Autodesk Inventor part; units mm, degrees
ref_plane "YZ Plane" through (0, 0, 0) normal (1, 0, 0) x (0, 1, 0)
ref_plane "XZ Plane" through (0, 0, 0) normal (0, 1, 0) x (-1, 0, 0)
ref_plane "XY Plane" through (0, 0, 0) normal (0, 0, 1) x (1, 0, 0)
sketch "Sketch1" plane through (0, 0, 0) normal (0, 0, 1) x (1, 0, 0)
  circle A0 centre (0, 0) radius 1.5
  dimension "Diameter" = 3
extrude "Extrusion1" add sketch "Sketch1" along normal blind 48
sketch "Sketch2" plane through (0, 0, 0) normal (0, 0, -1) x (-1, 0, 0)
  circle A0 centre (0, 0) radius 1.5 construction
  circle A1 centre (0, 0) radius 2.25
  dimension "Head_Washer_Diameter" = 4.5
extrude "Extrusion2" add sketch "Sketch2" along normal blind 0.25
sketch "Sketch3" plane through (0, 0, -0.25) normal (0, 0, -1) x (-1, 0, 0)
  circle A0 centre (0, 0) radius 2.25 construction
  line L0 (-2.25, 1.299) -> (0, 2.5981)
  line L1 (0, 2.5981) -> (2.25, 1.299)
  line L2 (2.25, 1.299) -> (2.25, -1.299)
  line L3 (2.25, -1.299) -> (0, -2.5981)
  line L4 (0, -2.5981) -> (-2.25, -1.299)
  line L5 (-2.25, -1.299) -> (-2.25, 1.299)
extrude "Extrusion3" add sketch "Sketch3" along normal blind 2.001
thread "Thread1"
chamfer "Chamfer1" distance 0.25 angle 45 1 edges at (-1.5, 0, 48)
sketch "Sketch4" plane through (0, 0, 0) normal (0, 1, 0) x (-1, 0, 0)
  line L0 (-2.25, -0.25) -> (-2.25, -2.251) construction
  line L1 (-2.25, -0.25) -> (-2.25, -2.251) construction
  line L2 (-2.25, -2.251) -> (-3.45, -2.251)
  line L3 (-3.45, -2.251) -> (-3.45, -1.5582)
  line L4 (-3.45, -1.5582) -> (-2.25, -2.251)
  line L5 (0, 0) -> (0, -6.83)
  point P0 (-2.25, -0.25)
  dimension "Head_Chamfer_Angle" = 30
  dimension "d14" = 1.2
revolve "Revolution1" cut sketch "Sketch4" angle 360 about axis through (0, 0, 0) along (0, 0, -1)
equation "\"Head_Washer_Diameter\" = 1.5 * Diameter"
equation "\"Head_Height\" = 0.667 * Diameter"
equation "\"d14\" = 0.4 * Diameter"
properties part number "Hex Head Cap Screw"
The listing builds one solid part. Answer for the finished solid, in the listing's coordinates (mm). A direction names the side the tool comes from. Round coordinates to 2 decimals unless told otherwise and drop trailing zeros. Order: outer loops, then holes, each group sorted by start corner. A loop starts at its lowest first (then second) coordinate and runs counter-clockwise, first axis right, second up. Notation, with made-up numbers: (-12, -32.75) -> (38, -32.75) arc R31 ccw to (38, -2.75) -> close; hole circle Ø2 at (71.5, -26). An arc over 180 degrees is marked (long way). One line per item, written item: value.
Item 1: Find section A-A, the plane z = 18.5. Give the vertices of the cut face in (x, y).
Taken from the geometry:
outline: circle Ø3 at (0, 0)
Item 2: Given P1, Ø0.5, axis at x = -0.5, y = 2.5, coming from the +Z side; P2, Ø0.6, axis at x = -2, y = -0.5, coming from the +Z side; P3, Ø3, axis at y = 1.5, z = 14.5, coming from the +X side, each flat-ended and moving along its own axis, determine where each tip first touches the part or whether it passes through.
Taken from the geometry:
P1: stops at z = -0.25
P2: stops at z = 0
P3: stops at x = 1.5
Item 3: For faces 1 (the conical face through (2.075, -1.205, -2.165)), 2 (the flat face through (2, 0, 0)), determine the directions among +Z, -Z, +X, -X, +Y, -Y from which every point of the face is accessible in a straight line to the end or side of a thin tool.
Taken from the geometry:
face 1: -Z, +X, -Y
face 2: +Z
Item 4: Straight lines are drawn through the part: L1, parallel to Z at x = -0.4, y = 1.9; L2, parallel to X at y = -0.25, z = 9.5; L3, parallel to X at y = 0.4, z = 25. For each, find the intervals that lie inside material, in ascending order.
Taken from the geometry:
L1: z = -2.25 to 0
L2: x = -1.48 to 1.48
L3: x = -1.45 to 1.45
